Check sheet for the modelled part. Datum: model origin and axes. Units: mm. A direction names the side the tool comes from. Round coordinates to 2 decimals unless told otherwise and drop trailing zeros. Loops run counter-clockwise (first coordinate to the right, second up) from the corner with the lowest first, then second, coordinate; pieces in that order, holes last. Notation, with made-up numbers: (-1, -23.75) - (13, -23.75) arc R34 cw to (13, 12.25) - close; hole circle Ø6 at (66, 8.25). An arc over 180 degrees is marked (long way). Put each result on its own line as item: value.
```python
from build123d import *

# Parameters (mm, degrees)
SKETCH1_R               = 12
SKETCH1_R_2             = 6.4
BOSS_EXTRUDE1_DEPTH     = 50
CUT_EXTRUDE1_DEPTH      = 53.80151513
CUT_EXTRUDE1_DEPTH_BACK = 53.80151513
SKETCH2_R               = 12
SKETCH2_R_2             = 8
BOSS_EXTRUDE2_DEPTH     = 50
SKETCH4_W               = 29
SKETCH4_H               = 42.03410999
CUT_EXTRUDE2_DEPTH      = 79.288280436
CUT_EXTRUDE6_DEPTH      = 79.288280436
CUT_EXTRUDE6_DEPTH_BACK = 79.288280436
SKETCH8_R               = 2.5
CUT_EXTRUDE9_START      = -10
CUT_EXTRUDE9_DEPTH      = 20
SKETCH10_W              = 3.2
SKETCH10_H              = 1.6
CUT_EXTRUDE10_DEPTH     = 20
FILLET1_R               = 10


with BuildPart() as part:
    # Sketch1 → Boss-Extrude1 (new body)
    with BuildSketch(Plane.XY):
        Circle(SKETCH1_R)
        Circle(SKETCH1_R_2, mode=Mode.SUBTRACT)
    extrude(amount=BOSS_EXTRUDE1_DEPTH)

    # Sketch2 → Cut-Extrude1 (cut, two sides: drawn at the far end of the back side and taken through both)
    with BuildSketch(Plane.XY.offset(50).offset(-CUT_EXTRUDE1_DEPTH_BACK)):
        Circle(SKETCH2_R)
        Circle(SKETCH2_R_2, mode=Mode.SUBTRACT)
    extrude(amount=CUT_EXTRUDE1_DEPTH + CUT_EXTRUDE1_DEPTH_BACK, mode=Mode.SUBTRACT)

    # Sketch3 → Boss-Extrude2 (add, through all)
    with BuildSketch(Plane.XY.offset(50)):
        with BuildLine():
            Line((-8, 0), (-8, -32))
            Line((-8, -32), (9.67766953, -49.67766953))
            Line((9.67766953, -49.67766953), (18, -49.67766953))
            Line((18, -49.67766953), (18, -47.076150072))
            Line((18, -47.076150072), (26.076150072, -47.076150072))
            Line((26.076150072, -47.076150072), (26.076150072, -35.076150072))
            Line((26.076150072, -35.076150072), (18, -35.076150072))
            Line((18, -35.076150072), (18, -28))
            Line((18, -28), (8, -28))
            Line((8, -28), (8, 0))
            ThreePointArc((8, 0), (0, -8), (-8, 0))
        make_face()
    extrude(amount=-BOSS_EXTRUDE2_DEPTH)

    # Sketch4 → Cut-Extrude2 (cut, through all)
    with BuildSketch(Plane(origin=(26.076150072, 0, 0), x_dir=(0, 0, -1), z_dir=(1, 0, 0))):
        with Locations((-25.5, -6.982945005)):
            Rectangle(SKETCH4_W, SKETCH4_H)
    extrude(amount=-CUT_EXTRUDE2_DEPTH, mode=Mode.SUBTRACT)

    # Sketch8 → Cut-Extrude6 (cut, two sides: drawn at the far end of the back side and taken through both)
    with BuildSketch(Plane(origin=(26.076150072, 0, 0), x_dir=(0, 0, -1), z_dir=(1, 0, 0)).offset(-CUT_EXTRUDE6_DEPTH_BACK)):
        with Locations(Location((-30.5, -41.076150072, 0), (0, 0, 90))):
            Circle(SKETCH8_R)
        with Locations(Location((-20.5, -41.076150072, 0), (0, 0, 90))):
            Circle(SKETCH8_R)
    extrude(amount=CUT_EXTRUDE6_DEPTH + CUT_EXTRUDE6_DEPTH_BACK, mode=Mode.SUBTRACT)

    # Sketch9 → Cut-Extrude9 (cut)
    with BuildSketch(Plane(origin=(26.076150072, 0, 0), x_dir=(0, 0, -1), z_dir=(1, 0, 0)).offset(CUT_EXTRUDE9_START)):
        with BuildLine():
            Line((-20.5, -36.076150072), (-30.5, -36.076150072))
            ThreePointArc((-30.5, -36.076150072), (-35.5, -41.076150072), (-30.5, -46.076150072))
            Line((-30.5, -46.076150072), (-20.5, -46.076150072))
            ThreePointArc((-20.5, -46.076150072), (-15.5, -41.076150072), (-20.5, -36.076150072))
        make_face()
    extrude(amount=-CUT_EXTRUDE9_DEPTH, mode=Mode.SUBTRACT)

    # Sketch10 → Cut-Extrude10 (cut)
    with BuildSketch(Plane(origin=(0, 0, 0), x_dir=(-1, 0, 0), z_dir=(0, 0, -1))):
        with Locations((0, -6.996773354)):
            Rectangle(SKETCH10_W, SKETCH10_H)
    extrude(amount=-CUT_EXTRUDE10_DEPTH, mode=Mode.SUBTRACT)

    # Fillet1
    # the kernel refuses this fillet: 10 mm, written as the material it adds along each edge
    with BuildSketch(Plane(origin=(8, -28, 11), x_dir=(0, 1, 0), z_dir=(0, 0, -1))) as fillet1_piece_1:
        with BuildLine():
            CenterArc((FILLET1_R, FILLET1_R), FILLET1_R, 180, 90)
            Line((0, FILLET1_R), (0, 0))
            Line((0, 0), (FILLET1_R, 0))
        make_face()
    extrude(amount=11)
    with BuildSketch(Plane(origin=(8, -28, 50), x_dir=(1, 0, 0), z_dir=(0, 0, -1))) as fillet1_piece_2:
        with BuildLine():
            CenterArc((FILLET1_R, -FILLET1_R), FILLET1_R, 90, 90)
            Line((0, -FILLET1_R), (0, 0))
            Line((0, 0), (FILLET1_R, 0))
        make_face()
    extrude(amount=10)
    # the kernel refuses this fillet: 10 mm, written as the material it takes off along each edge
    with BuildSketch(Plane(origin=(-8, -32, 60.355339059), x_dir=(0.7071067811865476, -0.7071067811865474, 0), z_dir=(0, 0, -1)), Plane(origin=(9.67766953, -49.67766953, 60.355339059), x_dir=(1, 0, 0), z_dir=(0, 0, -1))) as fillet1_2_piece_1:
        with BuildLine():
            CenterArc((FILLET1_R * 0.414213562373, -FILLET1_R), FILLET1_R, 90, 45)
            Line((-FILLET1_R * 0.292893218813, -FILLET1_R * 0.292893218813), (0, 0))
            Line((0, 0), (FILLET1_R * 0.414213562373, 0))
        make_face()
    extrude(amount=70.710678119, mode=Mode.SUBTRACT)


solid = part.part
```
Item 1: Section check C-C on z = 46. Enter the section's corners in (x, y).
Filled sheet:
outline: (-8, -27.86) arc R10 ccw to (-5.07, -34.93) - (6.75, -46.75) arc R10 ccw to (13.82, -49.68) - (18, -49.68) - (18, -47.08) - (26.08, -47.08) - (26.08, -35.08) - (18, -35.08) - (18, -28) arc R10 cw to (8, -18) - (8, 0) arc R8 ccw to (-8, 0) - close; hole circle Ø12.8 at (0, 0)
Item 2: Release check for a two-part mould opening along Z. For faces 4 (the cylindrical face through (8.44, -39.26, 35.16)), 5 (the flat face through (5, -27, 0)), 6 (the cylindrical face through (0, 8, 5)), 7 (the flat face through (5, -28, 50)) record: +Z half, -Z half, draft (parallel to the pull), parting line (faces both ways), or undercut.
Filled sheet:
face 4: undercut
face 5: -Z half
face 6: draft
face 7: +Z half
Item 3: Section check D-D on x = 15. Enter the section's corners in (y, z), then the cut area to 3 significant figures.
Filled sheet:
outline: (-49.68, 0) - (-27.54, 0) - (-27.54, 11) - (-28, 11) - (-28, 40) - (-27.54, 40) - (-27.54, 50) - (-49.68, 50) - close; hole (-46.08, 20.5) arc R5 ccw to (-36.08, 20.5) - (-36.08, 30.5) arc R5 ccw to (-46.08, 30.5) - close
area: 915 mm²
Item 4: Thickness scan on line 1 (X direction, y = 0, z = 42.25); line 2 (Z direction, x = 9.5, y = -24); line 3 (Y direction, x = 22, z = 20.5). Record the ranges inside material, lowest first. Write a range as from..to.
Filled sheet:
line 1: -8..-6.4, 6.4..8
line 2: 0..11, 40..50
line 3: -47.08..-43.58, -38.58..-35.08
Item 5: Go/stop test with flat-tipped pins: pin 1 (10 mm diameter, centred on x = 4.5, z = 22.5, fed in from -Y); pin 2 (8 mm diameter, centred on x = 8, z = 27.5, fed in from -Y); pin 3 (2.5 mm diameter, centred on x = 20, z = 32, fed in from -Y); pin 4 (2 mm diameter, centred on y = -48, z = 21.5, fed in from +X). Record where each tip stops, or that it passes through.
Filled sheet:
pin 1: y = -48.7
pin 2: y = -49.51
pin 3: y = -47.08
pin 4: x = 26.08
Item 6: Section check A-A on y = -15.5. Enter the section's corners in (x, z), then the cut area to 3 significant figures.
Filled sheet:
outline: (-8, 0) - (8, 0) - (8, 11) - (-8, 11) - close; (-8, 40) - (8, 40) - (8, 50) - (-8, 50) - close
area: 336 mm²
Item 7: Section check B-B on x = 24. Enter the section's corners in (y, z), then the cut area to 3 significant figures.
Filled sheet:
outline: (-47.08, 0) - (-35.08, 0) - (-35.08, 50) - (-47.08, 50) - close; hole circle Ø5 at (-41.08, 20.5); hole circle Ø5 at (-41.08, 30.5)
area: 561 mm²
Item 8: Tool access check on faces 1 (the flat face through (11, -46.076, 26)), 2 (the flat face through (-1, -14, 40)), 3 (the flat face through (0, -7.797, 5)). Record the directions out of +Z, -Z, +X, -X, +Y, -Y that give a thin tool (end or side, any length) a straight path to the whole face; none if there is none.
Filled sheet:
face 1: -X
face 2: +X, -X, +Y
face 3: -Z
